from build123d import *

# Parameters (mm, degrees)
ESBO_O1_W                                         = 25
ESBO_O1_H                                         = 25
RESSALTO_EXTRUS_O1_DEPTH                          = 60
ESBO_O2_R                                         = 5.1
CORTE_EXTRUS_O1_DEPTH                             = 61
ESBO_O3_R                                         = 11
CORTE_EXTRUS_O2_DEPTH                             = 3.2
FURO_ROSCADO_PARA_CONDU_TE_DE_M3X0_51_D           = 3.15
FURO_ROSCADO_PARA_CONDU_TE_DE_M3X0_51_DEPTH       = 6
FURO_ROSCADO_PARA_CONDU_TE_DE_M3X0_51_CSINK_D     = 3.766
FURO_ROSCADO_PARA_CONDU_TE_DE_M3X0_51_CSINK_ANGLE = 90
FURO_ROSCADO_PARA_CONDU_TE_DE_M3X0_51_TIP         = 0.946355475
REBAIXO_PARA_SHCS_M31_AT_2_COUNT                  = 2
REBAIXO_PARA_SHCS_M31_AT_2_PITCH                  = 16
REBAIXO_PARA_SHCS_M31_AT_3_COUNT                  = 2
REBAIXO_PARA_SHCS_M31_AT_3_PITCH                  = 16
REBAIXO_PARA_SHCS_M31_AT_4_COUNT                  = 2
REBAIXO_PARA_SHCS_M31_AT_4_PITCH                  = 22.627416998


with BuildPart() as part:
    # Esboço1 → Ressalto-extrusão1 (new body)
    with BuildSketch(Plane.XY):
        Rectangle(ESBO_O1_W, ESBO_O1_H)
    extrude(amount=RESSALTO_EXTRUS_O1_DEPTH)

    # Esboço2 → Corte-extrusão1 (cut, through all)
    with BuildSketch(Plane.XY.offset(60)):
        Circle(ESBO_O2_R)
    extrude(amount=-CORTE_EXTRUS_O1_DEPTH, mode=Mode.SUBTRACT)

    # Esboço3 → Corte-extrusão2 (cut)
    with BuildSketch(Plane.XY.offset(60)):
        Circle(ESBO_O3_R)
    extrude(amount=-CORTE_EXTRUS_O2_DEPTH, mode=Mode.SUBTRACT)

    # Furo roscado para conduíte de M3x0.51
    with Locations(Plane.XY.offset(56.8)):
        with Locations((0, 8), (8, 0), (0, -8), (-8, 0)):
            CounterSinkHole(FURO_ROSCADO_PARA_CONDU_TE_DE_M3X0_51_D / 2, FURO_ROSCADO_PARA_CONDU_TE_DE_M3X0_51_CSINK_D / 2, depth=FURO_ROSCADO_PARA_CONDU_TE_DE_M3X0_51_DEPTH, counter_sink_angle=FURO_ROSCADO_PARA_CONDU_TE_DE_M3X0_51_CSINK_ANGLE)
            with Locations((0, 0, -(FURO_ROSCADO_PARA_CONDU_TE_DE_M3X0_51_DEPTH + FURO_ROSCADO_PARA_CONDU_TE_DE_M3X0_51_TIP / 2))):  # 118° drill point
                Cone(0, FURO_ROSCADO_PARA_CONDU_TE_DE_M3X0_51_D / 2, FURO_ROSCADO_PARA_CONDU_TE_DE_M3X0_51_TIP, mode=Mode.SUBTRACT)

    # Esboço7 → Rebaixo para SHCS M31 (revolve, cut)
    with BuildSketch(Plane(origin=(-8, 12.5, 22), x_dir=(0, 0, 1), z_dir=(1, 0, 0))):
        Polygon((0, 0), (0, 25), (1.7, 25), (1.7, 3), (3.25, 3), (3.25, 0.025), (3.275, 0), align=None)
    rebaixo_para_shcs_m31 = revolve(axis=Axis((-8, 18.85, 22), (0, -1, 0)), mode=Mode.SUBTRACT)

    # Rebaixo para SHCS M31 at 2: Rebaixo para SHCS M31 ×2
    with Locations(*[(i * REBAIXO_PARA_SHCS_M31_AT_2_PITCH, 0, 0) for i in range(1, REBAIXO_PARA_SHCS_M31_AT_2_COUNT)]):
        add(rebaixo_para_shcs_m31, mode=Mode.SUBTRACT)

    # Rebaixo para SHCS M31 at 3: Rebaixo para SHCS M31 ×2
    with Locations(*[(0, 0, i * REBAIXO_PARA_SHCS_M31_AT_3_PITCH) for i in range(1, REBAIXO_PARA_SHCS_M31_AT_3_COUNT)]):
        add(rebaixo_para_shcs_m31, mode=Mode.SUBTRACT)

    # Rebaixo para SHCS M31 at 4: Rebaixo para SHCS M31 ×2
    with Locations(*[Vector(0.707106781, 0, 0.707106781) * (i * REBAIXO_PARA_SHCS_M31_AT_4_PITCH) for i in range(1, REBAIXO_PARA_SHCS_M31_AT_4_COUNT)]):
        add(rebaixo_para_shcs_m31, mode=Mode.SUBTRACT)


solid = part.part
Input: part model. Units: mm. Frame: model coordinates. A direction names the side the tool comes from. Give positions to 0.01 mm unless a question says otherwise; leave off trailing zeros. Loops run counter-clockwise (first coordinate to the right, second up) from the corner with the lowest first, then second, coordinate; pieces in that order, holes last. Notation, with made-up numbers: M 22.25,-14.75 L 60.25,-14.75 A19 cw 60.25,14.25 Z; hole C 6,78 d4. An arc over 180 degrees is marked long. Use CSV: the item, a comma, the result in double quotes.
(1) Pin query (flat end, axial travel): P1, Ø5.5, axis at x = 8, z = 22, coming from the +Y side; P2, Ø3, axis at x = 7, y = -5.5, coming from the +Z side. Return the tip coordinate at first contact, or that it passes through.
Outcome:
P1,"stops at y = 9.5"
P2,"stops at z = 56.8"
(2) Section A-A, the plane z = 38. Return loops of the section in (x, y) (3 decimals), plus the area to 3 significant figures.
Outcome:
outline,"M -12.5,-12.5 L -9.7,-12.5 L -9.7,9.5 L -11.25,9.5 L -11.25,12.475 L -11.275,12.5 L -12.5,12.5 Z; M -6.3,-12.5 L 6.3,-12.5 L 6.3,9.5 L 4.75,9.5 L 4.75,12.475 L 4.725,12.5 L -4.725,12.5 L -4.75,12.475 L -4.75,9.5 L -6.3,9.5 Z; M 9.7,-12.5 L 12.5,-12.5 L 12.5,12.5 L 11.275,12.5 L 11.25,12.475 L 11.25,9.5 L 9.7,9.5 Z; hole C 0,0 d10.2"
area,"355 mm²"
(3) Section B-B, the plane y = -3.5. Return loops of the section in (x, z).
Outcome:
outline,"M -12.5,0 L -3.71,0 L -3.71,56.8 L -10.43,56.8 L -10.43,60 L -12.5,60 Z; M 3.71,0 L 12.5,0 L 12.5,60 L 10.43,60 L 10.43,56.8 L 3.71,56.8 Z; hole C -8,22 d3.4; hole C -8,38 d3.4; hole C 8,22 d3.4; hole C 8,38 d3.4"
(4) Material intervals for L1, parallel to X at y = -6.75, z = 22; L2, parallel to Z at x = 8.25, y = 11.5; L3, parallel to Y at x = 0, z = 53.65 (3 decimals), sorted ascending. Write a range as [from, to].
Outcome:
L1,"x = [-12.5, -9.7], [-6.3, 6.3], [9.7, 12.5]"
L2,"z = [0, 18.76], [25.24, 34.76], [41.24, 60]"
L3,"y = [-12.5, -9.575], [-6.425, -5.1], [5.1, 6.425], [9.575, 12.5]"
(5) Set-up query: faces 1 (the face through (2, -5, 56.8)), 2 (the face through (-7.35, -1.35, 23.57)), 3 (the face through (9.4, 9.5, 36.6)). Return all of +Z, -Z, +X, -X, +Y, -Y with unobstructed straight access to the full face (end or side cutting, diameter ignored); none if empty.
Outcome:
face 1,"+Z"
face 2,"+Y, -Y"
face 3,"+Y"
(6) Pull-direction query (Z, two-part tool) for faces 4 (the face through (-6.6, 9.5, 20.6)), 5 (the face through (-12.5, 0, 30)), 6 (the face through (-0.202, -7.815, 50.018)); classes: pulls with the +Z half, pulls with the -Z half, needs draft (parallel to the pull), parting line crosses it, or undercut.
Outcome:
face 4,"undercut"
face 5,"needs draft"
face 6,"pulls with the +Z half"
(7) Section C-C, the plane x = -3.25. Return loops of the section in (y, z), plus the area to 3 significant figures.
Outcome:
outline,"M -12.5,0 L -3.93,0 L -3.93,56.8 L -10.51,56.8 L -10.51,60 L -12.5,60 Z; M 3.93,0 L 12.5,0 L 12.5,60 L 10.51,60 L 10.51,56.8 L 3.93,56.8 Z"
area,"986 mm²"
(8) Section D-D, the plane z = 31.5. Return loops of the section in (x, y), plus the area to 3 significant figures.
Outcome:
outline,"M -12.5,-12.5 L 12.5,-12.5 L 12.5,12.5 L -12.5,12.5 Z; hole C 0,0 d10.2"
area,"543 mm²"
